Source: CAD feature listing. Evaluate the final solid. Frame: model axes, mm. Face numbers are marked on the shaded views. A direction names the side the tool comes from. Round coordinates to 2 decimals unless told otherwise and drop trailing zeros. Order: outer loops, then holes, each group sorted by start corner. A loop starts at its lowest first (then second) coordinate and runs counter-clockwise, first axis right, second up. Notation, with made-up numbers: (37.5, 20.5) - (41.5, 20.5) arc R30 ccw to (41.5, 56.5) - close; hole circle Ø7 at (39.25, -39). An arc over 180 degrees is marked (long way). Put each result on its own line as item: value. Start each with the question number.
1) Section B-B on x = 0. Output: boundary loops of the cut face in (y, z), then the cut area to 3 significant figures.
2) Access query for the marked faces 1 and 2. Directions: +Z, -Z, +X, -X, +Y, -Y. A direction counts if a zero-diameter tool reaches every point of the face in a straight line with its end or side. Return the directions, or none.
3) Contact query for flat-ended pins moving along their axis: P1, Ø3, axis at y = 5, z = 2.5, coming from the +X side; P2, Ø4.5, axis at x = 5.5, z = 0, coming from the -Y side; P3, Ø1.2, axis at x = 6, z = -0.5, coming from the -Y side; P4, Ø3, axis at x = -2, y = 8, coming from the -Z side. Output: stop coordinate, or through.
4) Section D-D on y = 8.55. Output: boundary loops of the cut face in (x, z), then the cut area to 3 significant figures.
5) Section C-C on x = 5.5. Output: boundary loops of the cut face in (y, z).
6) Mould query, pull axis X, two halves, no side actions, for the marked faces 3, 4 and 5. Classes: +X half, -X half, draft (parallel to the pull), parting line (faces both ways), or undercut.
7) Line query: probe 1 along X at (y, z) = (4.95, 0); probe 2 along X at (y, z) = (8.3, 0); probe 3 along Y at (x, z) = (-8.75, -1.75). Output: solid intervals per line, ascending. Write a range as [from, to].
8) Section A-A on y = 5.7. Output: boundary loops of the cut face in (x, z) (3 decimals), then the cut area to 3 significant figures.
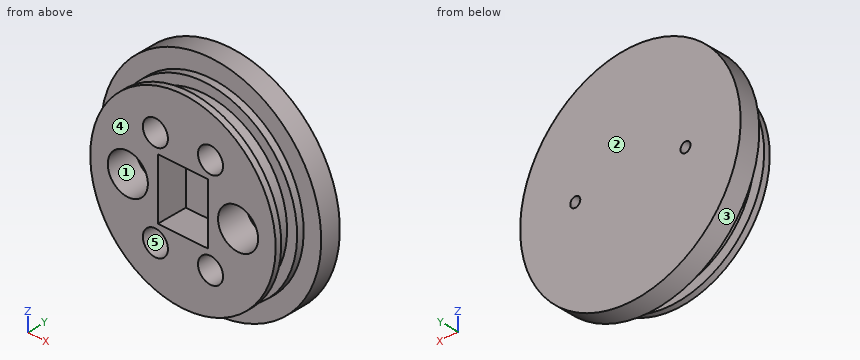
```python
from build123d import *

# Parameters (mm, degrees)
SKETCH_1_R           = 11
EXTRUDE_1_DEPTH      = 9
SKETCH_2_R           = 0.5
CUT_EXTRUDE_1_DEPTH  = 18.972200756
SKETCH_3_R           = 16.549134696
SKETCH_3_R_2         = 9.25
CUT_EXTRUDE_2_DEPTH  = 7
SKETCH_4_W           = 2
SKETCH_4_H           = 1.7
SKETCH_5_W           = 5
SKETCH_5_H           = 6
CUT_EXTRUDE_3_DEPTH  = 7
SKETCH_8_R           = 1.25
CUT_EXTRUDE_6_DEPTH  = 1.5
SKETCH_9_W           = 7
SKETCH_9_H           = 8
SKETCH_9_W_2         = 5
SKETCH_9_H_2         = 6
CUT_EXTRUDE_7_DEPTH  = 2
CHAMFER_1_SIZE       = 0.5
SKETCH_10_R          = 16.70563627
CUT_EXTRUDE_8_DEPTH  = 4
SKETCH_11_R          = 2
CUT_EXTRUDE_9_DEPTH  = 3
SKETCH_12_R          = 1.25
CUT_EXTRUDE_10_DEPTH = 3


with BuildPart() as part:
    # 草图1 → 凸台-拉伸1 (new body)
    with BuildSketch(Plane(origin=(0, 0, 0), x_dir=(1, 0, 0), z_dir=(0, 1, 0))):
        with Locations(Location((0, 0, 0), (0, 0, 270))):
            Circle(SKETCH_1_R)
    extrude(amount=EXTRUDE_1_DEPTH)

    # 草图2 → 切除-拉伸1 (cut, through all)
    with BuildSketch(Plane(origin=(0, 9, 0), x_dir=(1, 0, 0), z_dir=(0, 1, 0))):
        with Locations(Location((-5.5, 0, 0), (0, 0, 270))):
            Circle(SKETCH_2_R)
        with Locations(Location((5.5, 0, 0), (0, 0, 270))):
            Circle(SKETCH_2_R)
    extrude(amount=-CUT_EXTRUDE_1_DEPTH, mode=Mode.SUBTRACT)

    # 草图3 → 切除-拉伸2 (cut)
    with BuildSketch(Plane.XZ):
        Circle(SKETCH_3_R)
        with Locations(Location((0, 0, 0), (0, 0, 270))):
            Circle(SKETCH_3_R_2, mode=Mode.SUBTRACT)
    extrude(amount=-CUT_EXTRUDE_2_DEPTH, mode=Mode.SUBTRACT)

    # 草图4 → 切除-旋转1 (revolve, cut)
    with BuildSketch(Plane.XY, mode=Mode.PRIVATE) as cut_revolve_1_sk:
        with Locations((-9.25, 5.45)):
            Rectangle(SKETCH_4_W, SKETCH_4_H)
        with Locations((-9.25, 2.35)):
            Rectangle(SKETCH_4_W, SKETCH_4_H)
    revolve(cut_revolve_1_sk.sketch.rotate(Axis((0, 0, 0), (0, 1, 0)), 270), axis=Axis((0, 0, 0), (0, 1, 0)), mode=Mode.SUBTRACT)

    # 草图5 → 切除-拉伸3 (cut)
    with BuildSketch(Plane.XZ):
        Rectangle(SKETCH_5_W, SKETCH_5_H)
    extrude(amount=-CUT_EXTRUDE_3_DEPTH, mode=Mode.SUBTRACT)

    # 草图8 → 切除-拉伸6 (cut)
    with BuildSketch(Plane.XZ):
        with Locations(Location((-5.5, 0, 0), (0, 0, 270))):
            Circle(SKETCH_8_R)
        with Locations(Location((5.5, 0, 0), (0, 0, 270))):
            Circle(SKETCH_8_R)
    extrude(amount=-CUT_EXTRUDE_6_DEPTH, mode=Mode.SUBTRACT)

    # 草图9 → 切除-拉伸7 (cut)
    with BuildSketch(Plane.XZ):
        Rectangle(SKETCH_9_W, SKETCH_9_H)
        Rectangle(SKETCH_9_W_2, SKETCH_9_H_2, mode=Mode.SUBTRACT)
    extrude(amount=-CUT_EXTRUDE_7_DEPTH, mode=Mode.SUBTRACT)

    # 倒角1
    chamfer_1_edges = [part.edges().sort_by_distance(p)[0] for p in [
        (0, 0, 9.25),
    ]]
    chamfer(chamfer_1_edges, length=CHAMFER_1_SIZE)

    # 草图10 → 切除-拉伸8 (cut)
    with BuildSketch(Plane(origin=(0, 0, 0), x_dir=(-1, 0, 0), z_dir=(0, -1, 0))):
        Circle(SKETCH_10_R)
    extrude(amount=-CUT_EXTRUDE_8_DEPTH, mode=Mode.SUBTRACT)

    # 草图11 → 切除-拉伸9 (cut)
    with BuildSketch(Plane.XZ.offset(-4)):
        with Locations(Location((-5.5, 0, 0), (0, 0, 270))):
            Circle(SKETCH_11_R)
        with Locations(Location((5.5, 0, 0), (0, 0, 270))):
            Circle(SKETCH_11_R)
    extrude(amount=-CUT_EXTRUDE_9_DEPTH, mode=Mode.SUBTRACT)

    # 草图12 → 切除-拉伸10 (cut)
    with BuildSketch(Plane.XZ.offset(-4)):
        with Locations(Location((-2.75, 4.765, 0), (0, 0, 270))):
            Circle(SKETCH_12_R)
        with Locations(Location((2.75, 4.765, 0), (0, 0, 270))):
            Circle(SKETCH_12_R)
        with Locations(Location((2.75, -4.765, 0), (0, 0, 270))):
            Circle(SKETCH_12_R)
        with Locations(Location((-2.75, -4.765, 0), (0, 0, 270))):
            Circle(SKETCH_12_R)
    extrude(amount=-CUT_EXTRUDE_10_DEPTH, mode=Mode.SUBTRACT)


solid = part.part
```
Answer sheet:
1. outline: (4, -9.25) - (4.6, -9.25) - (4.6, -8.25) - (6.3, -8.25) - (6.3, -9.25) - (7, -9.25) - (7, -11) - (9, -11) - (9, 11) - (7, 11) - (7, 9.25) - (6.3, 9.25) - (6.3, 8.25) - (4.6, 8.25) - (4.6, 9.25) - (4, 9.25) - (4, 3) - (7, 3) - (7, -3) - (4, -3) - close
1. area: 78.1 mm^2
2. face 1: -Y
2. face 2: +Z, -Z, +X, -X, +Y
3. P1: x = 9.19
3. P2: y = 4
3. P3: y = 7
3. P4: z = -10.99
4. outline: circle Ø22 at (0, 0); hole circle Ø1 at (-5.5, 0); hole circle Ø1 at (5.5, 0)
4. area: 379 mm^2
5. outline: (4, -7.44) - (4.6, -7.44) - (4.6, -6.15) - (6.3, -6.15) - (6.3, -7.44) - (7, -7.44) - (7, -9.53) - (9, -9.53) - (9, -0.5) - (7, -0.5) - (7, -2) - (4, -2) - close; (4, 2) - (7, 2) - (7, 0.5) - (9, 0.5) - (9, 9.53) - (7, 9.53) - (7, 7.44) - (6.3, 7.44) - (6.3, 6.15) - (4.6, 6.15) - (4.6, 7.44) - (4, 7.44) - close
6. face 3: parting line
6. face 4: draft
6. face 5: undercut
7. probe 1: [-8.25, -7.5], [-3.5, -2.5], [2.5, 3.5], [7.5, 8.25]
7. probe 2: [-11, -6], [-5, 5], [6, 11]
7. probe 3: [4, 4.6], [6.3, 9]
8. outline: circle Ø16.5 at (0, 0); hole circle Ø4 at (-5.5, 0); hole circle Ø2.5 at (-2.75, -4.765); hole circle Ø2.5 at (-2.75, 4.765); hole (-2.5, -3) - (2.5, -3) - (2.5, 3) - (-2.5, 3) - close; hole circle Ø2.5 at (2.75, -4.765); hole circle Ø2.5 at (2.75, 4.765); hole circle Ø4 at (5.5, 0)
8. area: 139 mm^2
